Verification items for the finished model (mm, model axes). Give positions to 0.01 mm unless a question says otherwise; leave off trailing zeros. Order: outer loops, then holes, each group sorted by start corner. A loop starts at its lowest first (then second) coordinate and runs counter-clockwise, first axis right, second up. Notation, with made-up numbers: (-13, 31.5) - (12, 31.5) arc R14 ccw to (12, 44.5) - close; hole circle Ø9 at (16, 88.25). An arc over 180 degrees is marked (long way). Answer as a JSON object with one key per item and string values.
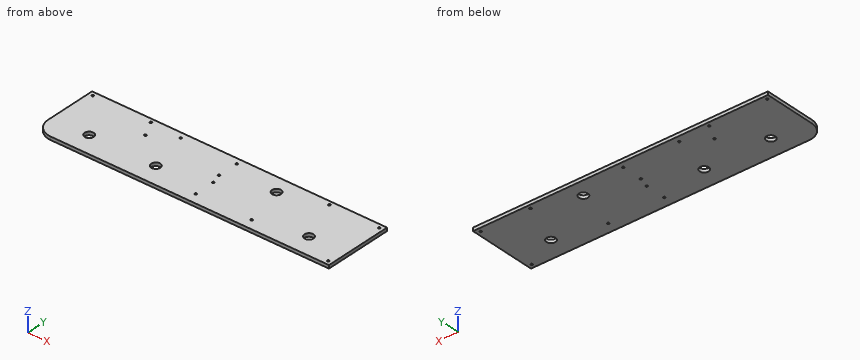
Autodesk Inventor part; units mm, degrees
ref_plane "YZ Plane" through (0, 0, 0) normal (1, 0, 0) x (0, 1, 0)
ref_plane "XZ Plane" through (0, 0, 0) normal (0, 1, 0) x (-1, 0, 0)
ref_plane "XY Plane" through (0, 0, 0) normal (0, 0, 1) x (1, 0, 0)
ref_plane "Work Plane1" through (-137.1271, 2.9342, 0.007) normal (0, 0, 1) x (-1, 0, 0)
sketch "Sketch1" plane through (-137.1271, 2.9342, 0.007) normal (0, 0, 1) x (-1, 0, 0)
  line L0 (6.35, -6.35) -> (-444.5, -6.35) construction
  line L1 (-444.5, -6.35) -> (-444.5, 98.6102) construction
  line L2 (6.35, -6.35) -> (-444.5, -6.35)
  line L3 (-444.5, -6.35) -> (-444.5, 98.6102)
  line L4 (-444.5, 98.6102) -> (-19.05, 98.6102)
  circle A0 centre (0, 0) radius 1.7 construction
  circle A1 centre (-101.6148, 24.9502) radius 1.7 construction
  circle A2 centre (-222.6743, 2.9342) radius 1.9304 construction
  circle A3 centre (-222.6743, 34.9382) radius 1.9304 construction
  circle A4 centre (-227.4763, 50.9282) radius 1.9304 construction
  circle A5 centre (-227.4763, 82.9322) radius 1.9304 construction
  circle A6 centre (-313.0743, 82.9322) radius 1.9304 construction
  circle A7 centre (-137.0763, 2.9342) radius 1.9304 construction
  circle A8 centre (-438.15, 0) radius 1.7 construction
  circle A9 centre (-438.15, 92.2602) radius 1.7 construction
  circle A10 centre (-387.1214, 66.8602) radius 4.83 construction
  circle A11 centre (-51.0689, 66.8602) radius 5.2798 construction
  circle A12 centre (-153.0753, 66.9332) radius 4.15 construction
  circle A13 centre (-297.0753, 18.9332) radius 4.83 construction
  circle A14 centre (0, 0) radius 1.65
  circle A15 centre (-101.6148, 24.9502) radius 1.65
  circle A16 centre (-438.15, 0) radius 1.65
  circle A17 centre (-438.15, 92.2602) radius 1.65
  circle A18 centre (-137.0763, 2.9342) radius 1.65
  circle A19 centre (-222.6743, 2.9342) radius 1.65
  circle A20 centre (-222.6743, 34.9382) radius 1.65
  circle A21 centre (-227.4763, 50.9282) radius 1.65
  circle A22 centre (-227.4763, 82.9322) radius 1.65
  circle A23 centre (-313.0743, 82.9322) radius 1.65
  circle A24 centre (-51.0689, 66.8602) radius 6.95
  circle A25 centre (-153.0753, 66.9332) radius 6.95
  circle A26 centre (-297.0753, 18.9332) radius 6.95
  circle A27 centre (-387.1214, 66.8602) radius 6.95
  line L5 (6.35, -6.35) -> (6.35, 73.2102)
  arc A28 (6.35, 73.2102) -> (-19.05, 98.6102) centre (-19.05, 73.2102) ccw
  point P0 (-137.1271, 2.9342)
  point P1 (6.35, 98.6102)
  dimension "M3Clearance" = 3.3
  dimension "d1" = 3.3
  dimension "d2" = 3.3
  dimension "d3" = 3.3
  dimension "d4" = 3.3
  dimension "d5" = 3.3
  dimension "d6" = 3.3
  dimension "d7" = 3.3
  dimension "d8" = 3.3
  dimension "d9" = 3.3
  dimension "BearingHole" = 13.9
  dimension "d11" = 13.9
  dimension "d12" = 13.9
  dimension "d13" = 13.9
  dimension "d20" = 25.4
extrude "Extrusion1" add sketch "Sketch1" along normal blind 5
sketch "Sketch2" plane through (-137.1271, 2.9342, 5.007) normal (0, 0, 1) x (1, 0, 0)
  circle A0 centre (88.9, 0) radius 1.7 construction
  circle A1 centre (361.95, 0) radius 1.7 construction
  circle A2 centre (88.9, 0) radius 1.65
  circle A3 centre (361.95, 0) radius 1.65
  point P0 (137.1271, -2.9342)
  dimension "d16" = 3.3
  dimension "d17" = 3.3
extrude "Extrusion2" cut sketch "Sketch2" against normal through all
equation "\"d1\" = M3Clearance"
equation "\"d2\" = M3Clearance"
equation "\"d3\" = M3Clearance"
equation "\"d4\" = M3Clearance"
equation "\"d5\" = M3Clearance"
equation "\"d6\" = M3Clearance"
equation "\"d7\" = M3Clearance"
equation "\"d8\" = M3Clearance"
equation "\"d9\" = M3Clearance"
equation "\"d16\" = M3Clearance"
equation "\"d17\" = M3Clearance"
properties part number "outside wall 2"
(1) Material ranges on line 1 along X through (y, z) = (3, 1.7); line 2 along Y through (x, z) = (-36, 1.75); line 3 along X through (y, z) = (-67, 0.65), recorded low to high. Write a range as [from, to].
Computed values:
{"line 1": "x = [-143.48, -138.78], [-135.48, -49.88], [-46.58, 223.17], [226.47, 299.37], [302.67, 307.37]", "line 2": "y = [-95.68, -23.59], [-20.44, 9.28]", "line 3": "x = [-143.48, -92.29], [-79.82, 9.68], [22.22, 243.76], [256.23, 307.37]"}
(2) Section check B-B (z = 1.5). Count the separate pieces of the cut face and the enclosed holes in it, then the cut area to 3 significant figures.
Computed values:
{"separate pieces": "1", "enclosed holes": "16", "area": "46,500 mm²"}
(3) Section check A-A (x = 162). Record the cut outline in (y, z).
Computed values:
{"outline": "(-95.68, 0.01) - (-22.64, 0.01) - (-22.64, 5.01) - (-95.68, 5.01) - close; (-9.36, 0.01) - (9.28, 0.01) - (9.28, 5.01) - (-9.36, 5.01) - close"}
